```python
from build123d import *

# Parameters (mm, degrees)
SKETCH_W        = 33.7
SKETCH_H        = 16.25
SKETCH_W_2      = 12.7
SKETCH_H_2      = 8.6
PAD_DEPTH       = 3.75
SKETCH001_W     = 33.7
SKETCH001_H     = 16.25
SKETCH001_W_2   = 25.6
SKETCH001_H_2   = 8.6
PAD001_DEPTH    = 6.3
FILLET_R        = 3.5
SKETCH002_R     = 1.5
POCKET_DEPTH    = 3.751
PAD002_DEPTH    = 27.2
SKETCH004_W     = 0.875
SKETCH004_H     = 17.15
POCKET001_DEPTH = 33.701
FILLET001_R     = 1


with BuildPart() as part:
    # Sketch → Pad (new body)
    with BuildSketch(Plane.XY):
        Rectangle(SKETCH_W, SKETCH_H)
        Rectangle(SKETCH_W_2, SKETCH_H_2, mode=Mode.SUBTRACT)
    extrude(amount=PAD_DEPTH)

    # Sketch001 (on Face10 of Pad) → Pad001 (join)
    with BuildSketch(Plane.XY.offset(3.75)):
        Rectangle(SKETCH001_W, SKETCH001_H)
        Rectangle(SKETCH001_W_2, SKETCH001_H_2, mode=Mode.SUBTRACT)
    extrude(amount=PAD001_DEPTH)

    # Fillet
    fillet_edges = [part.edges().sort_by_distance(p)[0] for p in [
        (-12.8, 4.3, 6.9),
        (12.8, 4.3, 6.9),
        (12.8, -4.3, 6.9),
        (-12.8, -4.3, 6.9),
        (-16.85, -8.125, 5.025),
        (-16.85, 8.125, 5.025),
        (16.85, -8.125, 5.025),
        (16.85, 8.125, 5.025),
    ]]
    fillet(fillet_edges, radius=FILLET_R)

    # Sketch002 (on Face18 of Fillet) → Pocket (cut, through all)
    with BuildSketch(Plane.XY.offset(3.75)):
        with Locations((-9.575, 0)):
            Circle(SKETCH002_R)
        with Locations((9.575, 0)):
            Circle(SKETCH002_R)
    extrude(amount=-POCKET_DEPTH, mode=Mode.SUBTRACT)

    # Sketch003 (on Face16 of Pocket) → Pad002 (join)
    with BuildSketch(Plane.XY.offset(10.05)):
        with BuildLine():
            Line((-16.85, -41.625), (16.85, -41.625))
            Line((16.85, -5.5), (16.85, -41.625))
            Line((16.85, -4.625), (16.85, -5.5))
            ThreePointArc((16.73886, -5.5), (16.822104, -5.066015), (16.85, -4.625))
            Line((16.73886, -5.5), (-16.73886, -5.5))
            ThreePointArc((-16.85, -4.625), (-16.822104, -5.066015), (-16.73886, -5.5))
            Line((-16.85, -4.625), (-16.85, -5.5))
            Line((-16.85, -5.5), (-16.85, -41.625))
        make_face()
    extrude(amount=-PAD002_DEPTH)

    # Sketch004 (on Face26 of Pad002) → Pocket001 (cut, through all)
    with BuildSketch(Plane.YZ.offset(16.85)):
        Polygon((-41.625, 3.85), (-39.225, 3.85), (-39.225, 7.55), (-8.725, 7.55), (-8.725, -14.65), (-39.225, -14.65), (-39.225, -10.95), (-41.625, -10.95), align=None)
        with Locations((-5.0625, -8.575)):
            Rectangle(SKETCH004_W, SKETCH004_H)
    extrude(amount=-POCKET001_DEPTH, mode=Mode.SUBTRACT)

    # Fillet001
    fillet001_edges = [part.edges().sort_by_distance(p)[0] for p in [
        (0, -8.725, 7.55),
        (0, -39.225, 7.55),
        (0, -5.5, -17.15),
        (0, -8.725, -14.65),
        (0, -41.625, 10.05),
        (0, -41.625, -17.15),
        (0, -41.625, -10.95),
        (0, -41.625, 3.85),
        (0, -39.225, 3.85),
        (0, -39.225, -10.95),
        (0, -5.5, 0),
    ]]
    fillet(fillet001_edges, radius=FILLET001_R)


solid = part.part
```
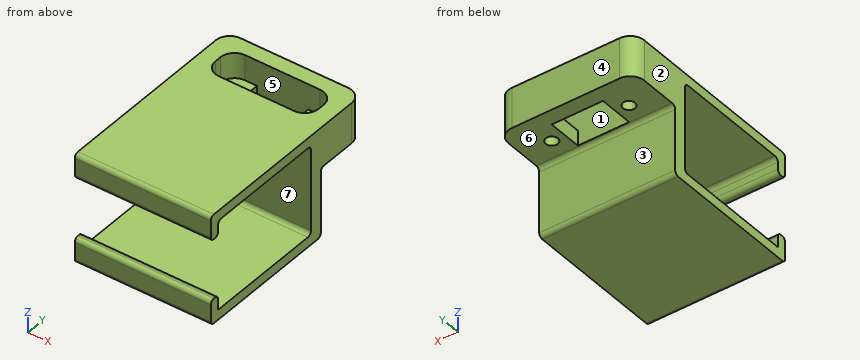
Can you work these out from the model? Positions are in its coordinate system, mm. Face numbers are marked on the shaded views. A direction names the side the tool comes from. Round coordinates to 2 decimals unless told otherwise and drop trailing zeros. Order: outer loops, then holes, each group sorted by start corner. A loop starts at its lowest first (then second) coordinate and runs counter-clockwise, first axis right, second up. Notation, with made-up numbers: (-32.5, 19.25) -> (13.5, 19.25) arc R30 ccw to (13.5, 52.25) -> close; hole circle Ø9 at (83.5, -6). An arc over 180 degrees is marked (long way). Return JSON: item names as keys, results as strings. Group by question number.
1. Which directions (+Z, -Z, +X, -X, +Y, -Y) give clear straight access to the entire face, cutting with the end or side of a thin tool? Please do the marked faces 4, 5, 6 and 7.
2. If we section it at B-B, the plane z = 2.25: Write out the boundary of the cut face in (x, y) (3 decimals).
3. We'd pull the mould along Y, two halves only. Please class the marked faces 1, 2 and 3: released by +Y, released by -Y, zero draft, split by the parting line, or undercut.
4. I need wall thicknesses on line 1 (Y direction, x = 7, z = 5.25) (3 decimals); line 2 (Z direction, x = 14, y = -30); line 3 (Y direction, x = 3.5, z = -12) (3 decimals). Which ranges of each line are inside material? Lowest first, please. Write a range as [from, to].
5. If we section it at A-A, the plane y = -36.5: Write out the boundary of the cut face in (x, z).
6. If we section it at D-D, the plane y = 0: Write out the boundary of the cut face in (x, z) (3 decimals).
7. Will these pins go through, and if not, where does the flat tip stop? pin 1 (7.5 mm diameter, centred on x = 6.5, z = -11.5, fed in from +Y); pin 2 (10 mm diameter, centred on x = 0, z = -0.5, fed in from -Y); pin 3 (3 mm diameter, centred on x = -8.5, y = 1, fed in from +Z); pin 4 (1 mm diameter, centred on y = -10.5, z = -10, fed in from +X).
Output values:
{
 "1": {"face 4": "+Z, -Z, +X, -X, +Y", "face 5": "+Z", "face 6": "-Z, +X, -X, +Y", "face 7": "+X, -X"},
 "2": {"outline": "(-16.85, -8.725) -> (16.85, -8.725) -> (16.85, 4.625) arc R3.5 ccw to (13.35, 8.125) -> (-13.35, 8.125) arc R3.5 ccw to (-16.85, 4.625) -> close; hole circle Ø3 at (-9.575, 0); hole (-6.35, -4.3) -> (6.35, -4.3) -> (6.35, 4.3) -> (-6.35, 4.3) -> close; hole circle Ø3 at (9.575, 0)"},
 "3": {"face 1": "undercut", "face 2": "zero draft", "face 3": "released by +Y"},
 "4": {"line 1": "[-41.625, -39.225], [-8.725, -4.3], [4.3, 8.125]", "line 2": "[-17.15, -14.65], [7.55, 10.05]", "line 3": "[-41.625, -39.225], [-8.725, -5.5]"},
 "5": {"outline": "(-16.85, -17.15) -> (16.85, -17.15) -> (16.85, -14.65) -> (-16.85, -14.65) -> close; (-16.85, 7.55) -> (16.85, 7.55) -> (16.85, 10.05) -> (-16.85, 10.05) -> close"},
 "6": {"outline": "(-16.85, 0) -> (-11.075, 0) -> (-11.075, 3.75) -> (-12.8, 3.75) -> (-12.8, 10.05) -> (-16.85, 10.05) -> close; (-8.075, 0) -> (-6.35, 0) -> (-6.35, 3.75) -> (-8.075, 3.75) -> close; (6.35, 0) -> (8.075, 0) -> (8.075, 3.75) -> (6.35, 3.75) -> close; (11.075, 0) -> (16.85, 0) -> (16.85, 10.05) -> (12.8, 10.05) -> (12.8, 3.75) -> (11.075, 3.75) -> close"},
 "7": {"pin 1": "y = -5.5", "pin 2": "y = -41.56", "pin 3": "z = 3.75", "pin 4": "through"}
}
